```python
from build123d import *

# Parameters (mm, degrees)
F0_W     = 20
F0_H     = 20
F1_DEPTH = 15
F1_TAPER = 3
F2_R     = 2
F4_DEPTH = 3


with BuildPart() as f1:
    # F0 (on Top) → F1 (new body)
    with BuildSketch(Plane.XY):
        with Locations((1.8707364798, -3.1114496091)):
            Rectangle(F0_W, F0_H)
    extrude(amount=F1_DEPTH, taper=F1_TAPER)

    # F2
    f2_edges = [f1.edges().sort_by_distance(p)[0] for p in [
        (-7.736205, 6.495492, 7.5),
        (1.870736, 6.102434, 15),
        (11.477678, 6.495492, 7.500009),
        (11.08462, -3.11145, 15),
        (11.477678, -12.718391, 7.5),
        (1.870736, -12.325333, 15),
        (-7.343147, -3.11145, 15),
        (-7.736205, -12.718391, 7.5),
    ]]
    fillet(f2_edges, radius=F2_R)

    # F3 (on face) → F4 (cut)
    with BuildSketch(Plane.XY.offset(15)):
        Polygon((2.8135806206, -2.1512166131), (1.8707364798, 3.426121315), (0.927892339, -2.1512166131), (-4.6021803282, -3.1114496091), (0.927892339, -4.071682605), (1.8707364798, -9.6490205332), (2.8135806206, -4.071682605), (8.3436532877, -3.1114496091), align=None)
    extrude(amount=-F4_DEPTH, mode=Mode.SUBTRACT)


solid = f1.part
```
Part model, mm, in its own coordinate system. A direction names the side the tool comes from. Give positions to 0.01 mm unless a question says otherwise; leave off trailing zeros. Loops run counter-clockwise (first coordinate to the right, second up) from the corner with the lowest first, then second, coordinate; pieces in that order, holes last. Notation, with made-up numbers: M 23.5,12 L 27.5,12 A26 ccw 27.5,40 Z; hole C 38.25,31 d8. An arc over 180 degrees is marked long. Return JSON: item names as keys, results as strings.
1) Saw through at B-B, the plane y = -7.5. List the corners of the cut face in (x, z).
Calculated:
{"outline": "M -8.13,0 L 11.87,0 L 11.18,13.1 A2 ccw 9.19,15 L 2.23,15 L 2.23,12 L 1.51,12 L 1.51,15 L -5.45,15 A2 ccw -7.44,13.1 Z"}
2) Pull direction Y, two halves, no side cores. Call faces 1 (the face through (-1.876, -3.585, 13.521)), 2 (the face through (1.768, 5.597, 14.436)), 3 (the face through (1.983, -12.773, 6.461)): released by +Y, released by -Y, zero draft, split by the parting line, or undercut.
Calculated:
{"face 1": "undercut", "face 2": "released by +Y", "face 3": "released by -Y"}
3) Saw through at C-C, the plane y = -2.5. List the corners of the cut face in (x, z), then the cut area to 3 significant figures.
Calculated:
{"outline": "M -8.13,0 L 11.87,0 L 11.18,13.1 A2 ccw 9.19,15 L 4.82,15 L 4.82,12 L -1.08,12 L -1.08,15 L -5.45,15 A2 ccw -7.44,13.1 Z", "area": "269 mm2"}
4) Saw through at A-A, the plane x = 8.75. List the corners of the cut face in (y, z), then the cut area to 3 significant figures.
Calculated:
{"outline": "M -13.11,0 L 6.89,0 L 6.2,13.1 A2 ccw 4.2,15 L -10.43,15 A2 ccw -12.42,13.1 Z", "area": "287 mm2"}
5) Flat gauge pins, fed straight in: pin 1 Ø1.5 at (x, z) = (7, 13) entering from +Y; pin 2 Ø2 at (y, z) = (-6, 12.5) entering from -X; pin 3 Ø5 at (y, z) = (-3.5, 13) entering from +X. Where does each tip first touch, or does it go through?
Calculated:
{"pin 1": "stops at y = 6.25", "pin 2": "stops at x = -7.53", "pin 3": "stops at x = 11.32"}
6) Drill centre lines: line 1 (Z direction, x = 1.25, y = -1); line 2 (Y direction, x = -5.5, z = 9.5); line 3 (X direction, y = -10.5, z = 13.25). Where is each one in solid material? Low to high.
Calculated:
{"line 1": "z = 0 to 12", "line 2": "y = -12.61 to 6.39", "line 3": "x = -7.43 to 11.17"}
7) 3-axis set-ups, long thin cutter, end or side, ignore diameter. For faces 4 (the face through (-6.837, -3.214, 14.436)), 5 (the face through (1.406, 0.676, 13.521)): which of +Z, -Z, +X, -X, +Y, -Y reach the whole face in a straight line?
Calculated:
{"face 4": "+Z, -X, +Y, -Y", "face 5": "+Z"}
